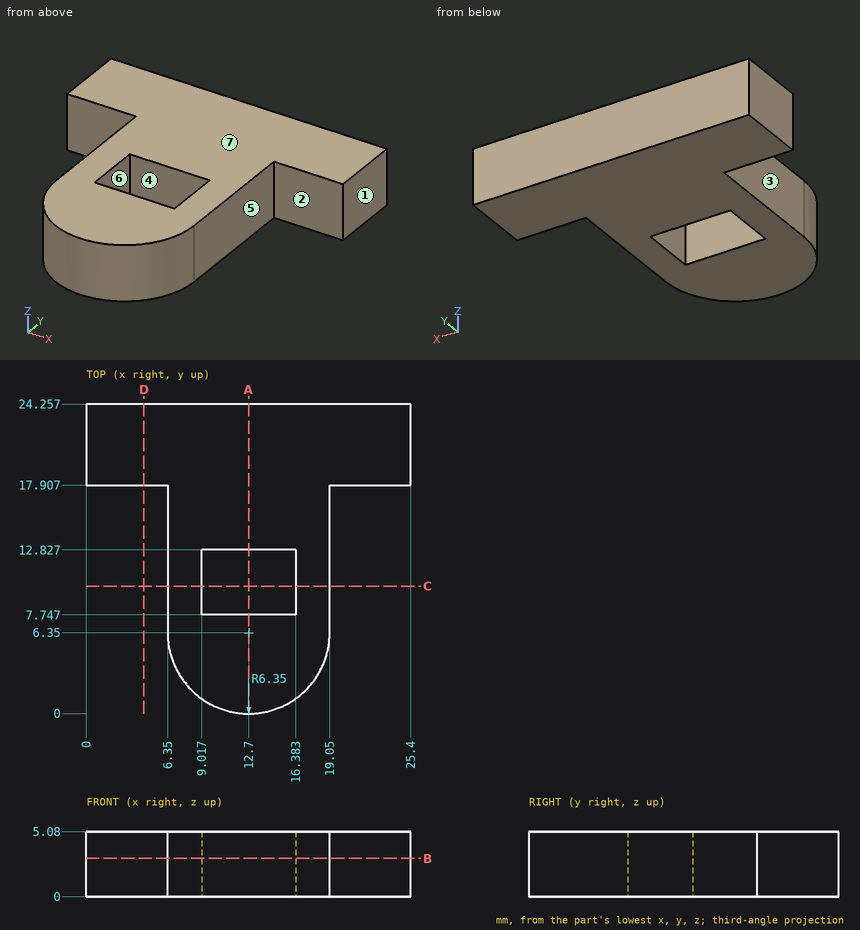
The drawing under review shows one solid part. Ordinate dimensions are in mm from its lowest x, y, z. A direction names the side the tool comes from. Round coordinates to 2 decimals unless told otherwise and drop trailing zeros. Loops run counter-clockwise (first coordinate to the right, second up) from the corner with the lowest first, then second, coordinate; pieces in that order, holes last. Notation, with made-up numbers: (-26.75, 21.5) - (-21.75, 21.5) arc R23 ccw to (-21.75, 31.5) - close; hole circle Ø8 at (24, 10.5). An arc over 180 degrees is marked (long way). One line per item, written item: value. Start each with the question number.
1) Consider section A-A on x = 12.7. Give the boundary of the cut face in (y, z), then the cut area to 3 significant figures.
2) For the marked faces 1, 2, 3 and 4, list the 3-axis set-ups (+Z, -Z, +X, -X, +Y, -Y) from which the entire face can be reached by the end or side of a thin tool; tool diameter is ignored.
3) To check wall thickness, follow L1, parallel to X at y = 9.5, z = 0.85; L2, parallel to Y at x = 19.5, z = 2.6; L3, parallel to X at y = 13, z = 2.35. State the ranges of each line that lie inside material, in increasing order. Write a range as from..to.
4) Draft analysis for pull direction X (two halves, no side actions). For the marked faces 5, 6 and 7, state which applies: +X half, -X half, draft (parallel to the pull), parting line (faces both ways), or undercut.
5) Consider section D-D on x = 4.5. Give the boundary of the cut face in (y, z).
6) Consider section B-B on z = 3. Give the boundary of the cut face in (x, y).
7) Insertion check: pin 1 Ø1.5 at (y, z) = (10, 3) entering from -X; pin 2 Ø1.5 at (y, z) = (13, 1.5) entering from +X; pin 3 Ø3 at (x, y) = (21, 14) entering from +Z. Each pin has a flat end and moves straight along its axis. Give the tip position at first contact, or say it passes through.
8) Consider section C-C on y = 10. Give the boundary of the cut face in (x, z), then the cut area to 3 significant figures.
Reported:
1. outline: (0, 0) - (7.75, 0) - (7.75, 5.08) - (0, 5.08) - close; (12.83, 0) - (24.26, 0) - (24.26, 5.08) - (12.83, 5.08) - close
1. area: 97.4 mm^2
2. face 1: +Z, -Z, +X, +Y, -Y
2. face 2: +Z, -Z, +X, -Y
2. face 3: +Z, -Z, -X, -Y
2. face 4: +Z, -Z
3. L1: x = 6.35..9.02, 16.38..19.05
3. L2: y = 17.91..24.26
3. L3: x = 6.35..19.05
4. face 5: +X half
4. face 6: undercut
4. face 7: draft
5. outline: (17.91, 0) - (24.26, 0) - (24.26, 5.08) - (17.91, 5.08) - close
6. outline: (0, 17.91) - (6.35, 17.91) - (6.35, 6.35) arc R6.35 ccw to (19.05, 6.35) - (19.05, 17.91) - (25.4, 17.91) - (25.4, 24.26) - (0, 24.26) - close; hole (9.02, 7.75) - (16.38, 7.75) - (16.38, 12.83) - (9.02, 12.83) - close
7. pin 1: stops at x = 6.35
7. pin 2: stops at x = 19.05
7. pin 3: passes through
8. outline: (6.35, 0) - (9.02, 0) - (9.02, 5.08) - (6.35, 5.08) - close; (16.38, 0) - (19.05, 0) - (19.05, 5.08) - (16.38, 5.08) - close
8. area: 27.1 mm^2
